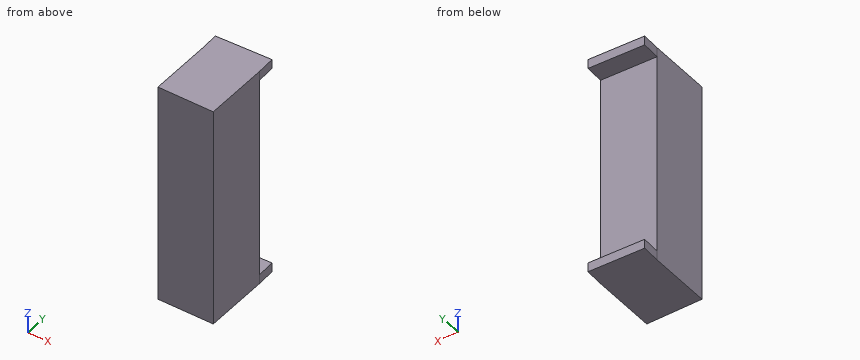
from build123d import *

# Parameters (mm, degrees)
SKETCH_1_W          = 30
SKETCH_1_H          = 120
EXTRUDE_1_DEPTH     = 35
CUT_EXTRUDE_1_DEPTH = 750.235385976
SKETCH_4_W          = 30.018286329
SKETCH_4_H          = 5
EXTRUDE_2_DEPTH     = 10


with BuildPart() as part:
    # Эскиз1 → Бобышка-Вытянуть1 (new body)
    with BuildSketch(Plane(origin=(708.734501427, 0, -6544.760847934), x_dir=(1, 0, 0), z_dir=(0, 1, 0))):
        with Locations((15, -60)):
            Rectangle(SKETCH_1_W, SKETCH_1_H)
    extrude(amount=EXTRUDE_1_DEPTH)

    # Эскиз3 → Вырез-Вытянуть1 (cut, through all)
    with BuildSketch(Plane.XY.offset(-6424.760847934)):
        Polygon((738.734501427, 35), (708.734501427, 33.952376915), (708.734501427, 35), align=None)
    extrude(amount=-CUT_EXTRUDE_1_DEPTH, mode=Mode.SUBTRACT)

    # Эскиз4 → Бобышка-Вытянуть2 (add)
    with BuildSketch(Plane(origin=(-0.320978232, 9.191613953, 0), x_dir=(0.9993908270190961, 0.03489949670249378, 0), z_dir=(-0.03489949670249378, 0.9993908270190961, 0))):
        with Locations((724.496823549, 6542.260847934)):
            Rectangle(SKETCH_4_W, SKETCH_4_H)
        with Locations((724.496823549, 6427.260847934)):
            Rectangle(SKETCH_4_W, SKETCH_4_H)
    extrude(amount=EXTRUDE_2_DEPTH)


solid = part.part
Here's how the part is built. I have some questions about the finished solid (model axes, mm). Give positions to 0.01 mm unless a question says otherwise; leave off trailing zeros. Loops run counter-clockwise (first coordinate to the right, second up) from the corner with the lowest first, then second, coordinate; pieces in that order, holes last. Notation, with made-up numbers: (-17, -35.5) -> (37, -35.5) arc R19 ccw to (37, -28.5) -> close; hole circle Ø4 at (48.25, 49.5). An arc over 180 degrees is marked (long way). Answer as a JSON object with one key per item and string values. Group by question number.
Item 1: I need wall thicknesses on L1, parallel to Z at x = 727, y = 36.5; L2, parallel to X at y = 11, z = -6533.5; L3, parallel to Y at x = 720, z = -6443. Which ranges of each line are inside material? Lowest first, please.
Item 2: Imagine slicing it at B-B on x = 733.5. Write out the boundary of the cut face in (y, z).
Item 3: Will these pins go through, and if not, where does the flat tip stop? pin 1 (5 mm diameter, centred on x = 730.5, z = -6470.5, fed in from +Y); pin 2 (1 mm diameter, centred on x = 734.5, z = -6465, fed in from +Y).
Item 4: Imagine slicing it at C-C on x = 718. Write out the boundary of the cut face in (y, z).
Item 5: Imagine slicing it at A-A on z = -6499. Write out the boundary of the cut face in (x, y), then the cut area to 3 significant figures.
Answer list:
{
 "1": {"L1": "z = -6544.76 to -6539.76, -6429.76 to -6424.76", "L2": "x = 708.73 to 738.73", "L3": "y = 0 to 34.35"},
 "2": {"outline": "(0, -6544.76) -> (44.82, -6544.76) -> (44.82, -6539.76) -> (34.82, -6539.76) -> (34.82, -6429.76) -> (44.82, -6429.76) -> (44.82, -6424.76) -> (0, -6424.76) -> close"},
 "3": {"pin 1": "stops at y = 34.8", "pin 2": "stops at y = 34.87"},
 "4": {"outline": "(0, -6544.76) -> (44.28, -6544.76) -> (44.28, -6539.76) -> (34.28, -6539.76) -> (34.28, -6429.76) -> (44.28, -6429.76) -> (44.28, -6424.76) -> (0, -6424.76) -> close"},
 "5": {"outline": "(708.73, 0) -> (738.73, 0) -> (738.73, 35) -> (708.73, 33.95) -> close", "area": "1,030 mm2"}
}
